```python
from build123d import *

# Parameters (mm, degrees)
SKETCH_1_W          = 70
SKETCH_1_H          = 50
EXTRUDE_1_DEPTH     = 50
SKETCH_2_R          = 15
EXTRUDE_2_DEPTH     = 10
SKETCH_3_R          = 10
CUT_EXTRUDE_1_DEPTH = 71
SKETCH_4_R          = 8
CUT_EXTRUDE_2_DEPTH = 35
SKETCH_5_R          = 2.5
CUT_EXTRUDE_3_DEPTH = 10


with BuildPart() as part:
    # 草图1 → 凸台-拉伸1 (new body)
    with BuildSketch(Plane(origin=(0, 0, 0), x_dir=(1, 0, 0), z_dir=(0, 1, 0))):
        Rectangle(SKETCH_1_W, SKETCH_1_H)
    extrude(amount=EXTRUDE_1_DEPTH)

    # 草图2 → 凸台-拉伸2 (add)
    with BuildSketch(Plane(origin=(0, 50, 0), x_dir=(1, 0, 0), z_dir=(0, 1, 0))):
        with Locations(Location((0, 0, 0), (0, 0, 270))):
            Circle(SKETCH_2_R)
    extrude(amount=EXTRUDE_2_DEPTH)

    # 草图3 → 切除-拉伸1 (cut, symmetric)
    with BuildSketch(Plane(origin=(0, 0, 0), x_dir=(0, 0, -1), z_dir=(1, 0, 0))):
        with Locations((0, 25)):
            Circle(SKETCH_3_R)
    extrude(amount=CUT_EXTRUDE_1_DEPTH, both=True, mode=Mode.SUBTRACT)

    # 草图4 → 切除-拉伸2 (cut)
    with BuildSketch(Plane(origin=(0, 60, 0), x_dir=(1, 0, 0), z_dir=(0, 1, 0))):
        with Locations(Location((0, 0, 0), (0, 0, 270))):
            Circle(SKETCH_4_R)
    extrude(amount=-CUT_EXTRUDE_2_DEPTH, mode=Mode.SUBTRACT)

    # 草图5 → 切除-拉伸3 (cut)
    with BuildSketch(Plane.XY.offset(25)):
        with Locations((-18, 25)):
            Circle(SKETCH_5_R)
        with Locations((18, 25)):
            Circle(SKETCH_5_R)
        with Locations((-18, 43)):
            Circle(SKETCH_5_R)
        with Locations((18, 43)):
            Circle(SKETCH_5_R)
    extrude(amount=-CUT_EXTRUDE_3_DEPTH, mode=Mode.SUBTRACT)


solid = part.part
```
CAD build for the part. Positions are in the model's coordinates, mm. A direction names the side the tool comes from. Round coordinates to 2 decimals unless told otherwise and drop trailing zeros. Write each loop counter-clockwise with the first axis right and the second up, starting at its lowest first coordinate (ties: lowest second). Pieces come first, ordered by that corner, then holes. Notation, with made-up numbers: (-40, 70.5) -> (-5, 70.5) arc R15 cw to (-5, 98.5) -> close; hole circle Ø9 at (33, 64). An arc over 180 degrees is marked (long way). Answer in a Markdown table with one row per item. Add a question column.
Item 1: Saw through at B-B, the plane x = 18. Write the cut outline in (y, z), then the cut area to 3 significant figures.
Item 2: Drill centre lines: line 1 (Y direction, x = 18, z = 18); line 2 (Y direction, x = -9.5, z = -0.5); line 3 (Z direction, x = 0, y = 46.75). Where is each one in solid material? Low to high. Write a range as from..to.
Item 3: Mould opens along Y. For faces 1 (the face through (18, 25, 15)), 2 (the face through (0, 0, 0)), 3 (the face through (-16, 50, 0)) say: pulls with the +Y half, pulls with the -Y half, needs draft (parallel to the pull), parting line crosses it, or undercut.
Item 4: Saw through at C-C, the plane y = 43. Write the cut outline in (x, z).
Item 5: Drop flat-ended pins along their axis: pin 1 Ø10 at (x, z) = (14, -15) entering from +Y; pin 2 Ø1.5 at (x, y) = (18.5, 25.5) entering from +Z; pin 3 Ø16 at (y, z) = (25, 0) entering from +X; pin 4 Ø18.5 at (x, z) = (0, 0) entering from +Y. Give the stop position or say it passes through.
Item 6: Saw through at A-A, the plane z = 0. Write the cut outline in (x, y).
Item 7: Which spindle directions (+Z, -Z, +X, -X, +Y, -Y) get a long thin tool onto all of the face, cutting with end or side? Do faces 4 (the face through (0, 25, -25)), 5 (the face through (-18, 43, 15)), 6 (the face through (-7.81, 45.7, -1.73)). Say none if no direction does.
Item 8: Saw through at D-D, the plane z = 20. Write the cut outline in (x, y).
Findings below:
| question | item | result |
|---|---|---|
| 1 | outline | (0, -25) -> (50, -25) -> (50, 25) -> (45.5, 25) -> (45.5, 15) -> (40.5, 15) -> (40.5, 25) -> (27.5, 25) -> (27.5, 15) -> (22.5, 15) -> (22.5, 25) -> (0, 25) -> close; hole circle Ø20 at (25, 0) |
| 1 | area | 2,090 mm^2 |
| 2 | line 1 | y = 0..22.5, 27.5..40.5, 45.5..50 |
| 2 | line 2 | y = 0..15.01, 34.99..60 |
| 2 | line 3 | z = -25..-8, 8..25 |
| 3 | face 1 | undercut |
| 3 | face 2 | pulls with the -Y half |
| 3 | face 3 | pulls with the +Y half |
| 4 | outline | (-35, -25) -> (35, -25) -> (35, 25) -> (20.5, 25) -> (20.5, 15) -> (15.5, 15) -> (15.5, 25) -> (-15.5, 25) -> (-15.5, 15) -> (-20.5, 15) -> (-20.5, 25) -> (-35, 25) -> close; hole circle Ø16 at (0, 0) |
| 5 | pin 1 | stops at y = 50 |
| 5 | pin 2 | stops at z = 15 |
| 5 | pin 3 | passes through |
| 5 | pin 4 | stops at y = 60 |
| 6 | outline | (-35, 0) -> (35, 0) -> (35, 15) -> (-35, 15) -> close; (-35, 35) -> (-8, 35) -> (-8, 60) -> (-15, 60) -> (-15, 50) -> (-35, 50) -> close; (8, 35) -> (35, 35) -> (35, 50) -> (15, 50) -> (15, 60) -> (8, 60) -> close |
| 7 | face 4 | -Z, +X, -X, +Y, -Y |
| 7 | face 5 | +Z |
| 7 | face 6 | +Y |
| 8 | outline | (-35, 0) -> (35, 0) -> (35, 50) -> (-35, 50) -> close; hole circle Ø5 at (-18, 25); hole circle Ø5 at (-18, 43); hole circle Ø5 at (18, 25); hole circle Ø5 at (18, 43) |
